Verification items for the finished model (mm, model axes). Face numbers are marked on the shaded views. A direction names the side the tool comes from. Give positions to 0.01 mm unless a question says otherwise; leave off trailing zeros. Order: outer loops, then holes, each group sorted by start corner. A loop starts at its lowest first (then second) coordinate and runs counter-clockwise, first axis right, second up.
from build123d import *

# Parameters (mm, degrees)
F1_DEPTH = 6.35


with BuildPart() as f1:
    # F0 (on Front) → F1 (new body)
    with BuildSketch(Plane.XZ):
        with BuildLine():
            ThreePointArc((11.4914766139, 0.1410518603), (11.4921258391, 0.0705272582), (11.4923422502, 0))
            ThreePointArc((11.4923422502, 0), (11.4921258391, -0.0705272582), (11.4914766139, -0.1410518603))
            Line((11.4914766139, -0.1410518603), (11.5924987112, 0))
            Line((11.5924987112, 0), (11.4914766139, 0.1410518603))
        make_face()
        with BuildLine():
            ThreePointArc((10.4146627839, 4.8588815063), (11.204205236, 2.5572867309), (11.4914766139, 0.1410518603))
            Line((11.4914766139, 0.1410518603), (11.5924987112, 0))
            Line((11.5924987112, 0), (13.8578264949, 3.1629584667))
            Line((13.8578264949, 3.1629584667), (10.44448044, 5.0297966865))
            Line((10.44448044, 5.0297966865), (10.4146627839, 4.8588815063))
        make_face()
        with BuildLine():
            Line((11.5924987112, 0), (11.4914766139, -0.1410518603))
            ThreePointArc((11.4914766139, -0.1410518603), (11.204205236, -2.5572867309), (10.4146627839, -4.8588815063))
            Line((10.4146627839, -4.8588815063), (10.44448044, -5.0297966865))
            Line((10.44448044, -5.0297966865), (13.8578264949, -3.1629584667))
            Line((13.8578264949, -3.1629584667), (11.5924987112, 0))
        make_face()
        with BuildLine():
            ThreePointArc((10.2922625668, 5.1130481761), (10.3542425867, 4.9863404267), (10.4146627839, 4.8588815063))
            Line((10.4146627839, 4.8588815063), (10.44448044, 5.0297966865))
            Line((10.44448044, 5.0297966865), (10.2922625668, 5.1130481761))
        make_face()
        with BuildLine():
            Line((10.44448044, -5.0297966865), (10.4146627839, -4.8588815063))
            ThreePointArc((10.4146627839, -4.8588815063), (10.3542425867, -4.9863404267), (10.2922625668, -5.1130481761))
            Line((10.2922625668, -5.1130481761), (10.44448044, -5.0297966865))
        make_face()
        with BuildLine():
            ThreePointArc((7.2750972621, 8.8964538004), (8.9850749785, 7.1653581925), (10.2922625668, 5.1130481761))
            Line((10.2922625668, 5.1130481761), (10.44448044, 5.0297966865))
            Line((10.44448044, 5.0297966865), (11.1131140025, 8.8624126846))
            Line((11.1131140025, 8.8624126846), (7.2278047245, 9.0633804529))
            Line((7.2278047245, 9.0633804529), (7.2750972621, 8.8964538004))
        make_face()
        with BuildLine():
            Line((10.44448044, -5.0297966865), (10.2922625668, -5.1130481761))
            ThreePointArc((10.2922625668, -5.1130481761), (8.9850749785, -7.1653581925), (7.2750972621, -8.8964538004))
            Line((7.2750972621, -8.8964538004), (7.2278047245, -9.0633804529))
            Line((7.2278047245, -9.0633804529), (11.1131140025, -8.8624126846))
            Line((11.1131140025, -8.8624126846), (10.44448044, -5.0297966865))
        make_face()
        with BuildLine():
            ThreePointArc((7.054539692, 9.0723425932), (7.1653581925, 8.9850749785), (7.2750972621, 8.8964538004))
            Line((7.2750972621, 8.8964538004), (7.2278047245, 9.0633804529))
            Line((7.2278047245, 9.0633804529), (7.054539692, 9.0723425932))
        make_face()
        with BuildLine():
            Line((7.2278047245, -9.0633804529), (7.2750972621, -8.8964538004))
            ThreePointArc((7.2750972621, -8.8964538004), (7.1653581925, -8.9850749785), (7.054539692, -9.0723425932))
            Line((7.054539692, -9.0723425932), (7.2278047245, -9.0633804529))
        make_face()
        with BuildLine():
            ThreePointArc((2.6946095043, 11.1719743114), (4.9863404267, 10.3542425867), (7.054539692, 9.0723425932))
            Line((7.054539692, 9.0723425932), (7.2278047245, 9.0633804529))
            Line((7.2278047245, 9.0633804529), (6.1673129885, 12.80655738))
            Line((6.1673129885, 12.80655738), (2.5795736401, 11.3018505655))
            Line((2.5795736401, 11.3018505655), (2.6946095043, 11.1719743114))
        make_face()
        with BuildLine():
            Line((7.2278047245, -9.0633804529), (7.054539692, -9.0723425932))
            ThreePointArc((7.054539692, -9.0723425932), (4.9863404267, -10.3542425867), (2.6946095043, -11.1719743114))
            Line((2.6946095043, -11.1719743114), (2.5795736401, -11.3018505655))
            Line((2.5795736401, -11.3018505655), (6.1673129885, -12.80655738))
            Line((6.1673129885, -12.80655738), (7.2278047245, -9.0633804529))
        make_face()
        with BuildLine():
            ThreePointArc((2.419578713, 11.2347482948), (2.5572867309, 11.204205236), (2.6946095043, 11.1719743114))
            Line((2.6946095043, 11.1719743114), (2.5795736401, 11.3018505655))
            Line((2.5795736401, 11.3018505655), (2.419578713, 11.2347482948))
        make_face()
        with BuildLine():
            Line((2.5795736401, -11.3018505655), (2.6946095043, -11.1719743114))
            ThreePointArc((2.6946095043, -11.1719743114), (2.5572867309, -11.204205236), (2.419578713, -11.2347482948))
            Line((2.419578713, -11.2347482948), (2.5795736401, -11.3018505655))
        make_face()
        with BuildLine():
            ThreePointArc((-2.419578713, 11.2347482948), (0, 11.4923422502), (2.419578713, 11.2347482948))
            Line((2.419578713, 11.2347482948), (2.5795736401, 11.3018505655))
            Line((2.5795736401, 11.3018505655), (0, 14.2142063241))
            Line((0, 14.2142063241), (-2.5795736401, 11.3018505655))
            Line((-2.5795736401, 11.3018505655), (-2.419578713, 11.2347482948))
        make_face()
        with BuildLine():
            Line((2.5795736401, -11.3018505655), (2.419578713, -11.2347482948))
            ThreePointArc((2.419578713, -11.2347482948), (0, -11.4923422502), (-2.419578713, -11.2347482948))
            Line((-2.419578713, -11.2347482948), (-2.5795736401, -11.3018505655))
            Line((-2.5795736401, -11.3018505655), (0, -14.2142063241))
            Line((0, -14.2142063241), (2.5795736401, -11.3018505655))
        make_face()
        with BuildLine():
            ThreePointArc((-2.6946095043, 11.1719743114), (-2.5572867309, 11.204205236), (-2.419578713, 11.2347482948))
            Line((-2.419578713, 11.2347482948), (-2.5795736401, 11.3018505655))
            Line((-2.5795736401, 11.3018505655), (-2.6946095043, 11.1719743114))
        make_face()
        with BuildLine():
            Line((-2.5795736401, -11.3018505655), (-2.419578713, -11.2347482948))
            ThreePointArc((-2.419578713, -11.2347482948), (-2.5572867309, -11.204205236), (-2.6946095043, -11.1719743114))
            Line((-2.6946095043, -11.1719743114), (-2.5795736401, -11.3018505655))
        make_face()
        with BuildLine():
            ThreePointArc((-7.054539692, 9.0723425932), (-4.9863404267, 10.3542425867), (-2.6946095043, 11.1719743114))
            Line((-2.6946095043, 11.1719743114), (-2.5795736401, 11.3018505655))
            Line((-2.5795736401, 11.3018505655), (-6.1673129885, 12.80655738))
            Line((-6.1673129885, 12.80655738), (-7.2278047245, 9.0633804529))
            Line((-7.2278047245, 9.0633804529), (-7.054539692, 9.0723425932))
        make_face()
        with BuildLine():
            Line((-2.5795736401, -11.3018505655), (-2.6946095043, -11.1719743114))
            ThreePointArc((-2.6946095043, -11.1719743114), (-4.9863404267, -10.3542425867), (-7.054539692, -9.0723425932))
            Line((-7.054539692, -9.0723425932), (-7.2278047245, -9.0633804529))
            Line((-7.2278047245, -9.0633804529), (-6.1673129885, -12.80655738))
            Line((-6.1673129885, -12.80655738), (-2.5795736401, -11.3018505655))
        make_face()
        with BuildLine():
            ThreePointArc((-7.2750972621, 8.8964538004), (-7.1653581925, 8.9850749785), (-7.054539692, 9.0723425932))
            Line((-7.054539692, 9.0723425932), (-7.2278047245, 9.0633804529))
            Line((-7.2278047245, 9.0633804529), (-7.2750972621, 8.8964538004))
        make_face()
        with BuildLine():
            Line((-7.2278047245, -9.0633804529), (-7.054539692, -9.0723425932))
            ThreePointArc((-7.054539692, -9.0723425932), (-7.1653581925, -8.9850749785), (-7.2750972621, -8.8964538004))
            Line((-7.2750972621, -8.8964538004), (-7.2278047245, -9.0633804529))
        make_face()
        with BuildLine():
            ThreePointArc((-10.2922625668, 5.1130481761), (-8.9850749785, 7.1653581925), (-7.2750972621, 8.8964538004))
            Line((-7.2750972621, 8.8964538004), (-7.2278047245, 9.0633804529))
            Line((-7.2278047245, 9.0633804529), (-11.1131140025, 8.8624126846))
            Line((-11.1131140025, 8.8624126846), (-10.44448044, 5.0297966865))
            Line((-10.44448044, 5.0297966865), (-10.2922625668, 5.1130481761))
        make_face()
        with BuildLine():
            Line((-7.2278047245, -9.0633804529), (-7.2750972621, -8.8964538004))
            ThreePointArc((-7.2750972621, -8.8964538004), (-8.9850749785, -7.1653581925), (-10.2922625668, -5.1130481761))
            Line((-10.2922625668, -5.1130481761), (-10.44448044, -5.0297966865))
            Line((-10.44448044, -5.0297966865), (-11.1131140025, -8.8624126846))
            Line((-11.1131140025, -8.8624126846), (-7.2278047245, -9.0633804529))
        make_face()
        with BuildLine():
            ThreePointArc((-10.4146627839, 4.8588815063), (-10.3542425867, 4.9863404267), (-10.2922625668, 5.1130481761))
            Line((-10.2922625668, 5.1130481761), (-10.44448044, 5.0297966865))
            Line((-10.44448044, 5.0297966865), (-10.4146627839, 4.8588815063))
        make_face()
        with BuildLine():
            Line((-10.44448044, -5.0297966865), (-10.2922625668, -5.1130481761))
            ThreePointArc((-10.2922625668, -5.1130481761), (-10.3542425867, -4.9863404267), (-10.4146627839, -4.8588815063))
            Line((-10.4146627839, -4.8588815063), (-10.44448044, -5.0297966865))
        make_face()
        with BuildLine():
            ThreePointArc((-11.4914766139, 0.1410518603), (-11.204205236, 2.5572867309), (-10.4146627839, 4.8588815063))
            Line((-10.4146627839, 4.8588815063), (-10.44448044, 5.0297966865))
            Line((-10.44448044, 5.0297966865), (-13.8578264949, 3.1629584667))
            Line((-13.8578264949, 3.1629584667), (-11.5924987112, 0))
            Line((-11.5924987112, 0), (-11.4914766139, 0.1410518603))
        make_face()
        with BuildLine():
            Line((-10.44448044, -5.0297966865), (-10.4146627839, -4.8588815063))
            ThreePointArc((-10.4146627839, -4.8588815063), (-11.204205236, -2.5572867309), (-11.4914766139, -0.1410518603))
            Line((-11.4914766139, -0.1410518603), (-11.5924987112, 0))
            Line((-11.5924987112, 0), (-13.8578264949, -3.1629584667))
            Line((-13.8578264949, -3.1629584667), (-10.44448044, -5.0297966865))
        make_face()
        with BuildLine():
            ThreePointArc((-11.4914766139, -0.1410518603), (-11.4923422502, 0), (-11.4914766139, 0.1410518603))
            Line((-11.4914766139, 0.1410518603), (-11.5924987112, 0))
            Line((-11.5924987112, 0), (-11.4914766139, -0.1410518603))
        make_face()
    extrude(amount=F1_DEPTH)


solid = f1.part
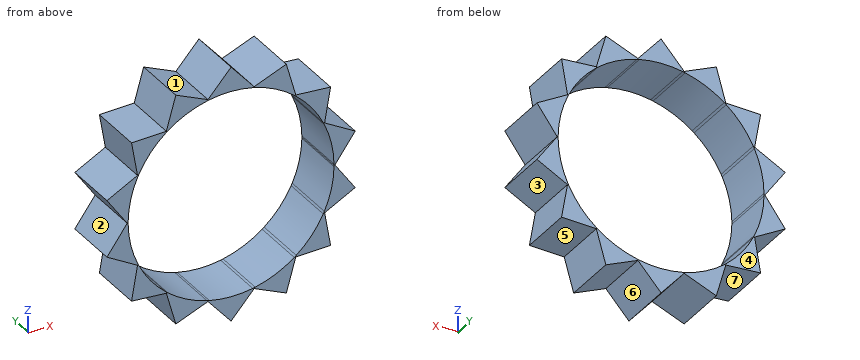
(1) Section check A-A, the plane x = -0.5. Enter the section's corners in (y, z), then the cut area to 3 significant figures.
Solved:
outline: (-6.35, -13.65) - (0, -13.65) - (0, -11.48) - (-6.35, -11.48) - close; (-6.35, 11.48) - (0, 11.48) - (0, 13.65) - (-6.35, 13.65) - close
area: 27.5 mm2
(2) Release check for a two-part mould opening along X. For the marked faces 4, 5, 6 and 7 record: pulls with the +X half, pulls with the -X half, needs draft (parallel to the pull), parting line crosses it, or undercut.
Solved:
face 4: needs draft
face 5: pulls with the +X half
face 6: undercut
face 7: pulls with the -X half
(3) Scan lines: line 1 (X direction, y = -3.25, z = 12.25) (3 decimals); line 2 (Z direction, x = -4, y = -3); line 3 (X direction, y = -2.25, z = -10.5). Record each from-to range of solid material in increasing order.
Solved:
line 1: x = -6.325 to -4.84, -1.74 to 1.74, 4.84 to 6.325
line 2: z = -11.9 to -10.77, 10.77 to 11.9
line 3: x = -6.82 to -4.67, 4.67 to 6.82
(4) Set-up check for the marked faces 1, 2 and 3: record each of +Z, -Z, +X, -X, +Y, -Y from which the full face is reachable in a straight line by a thin tool's end or side.
Solved:
face 1: +Z, +Y, -Y
face 2: -X, +Y, -Y
face 3: +X, +Y, -Y
(5) Section check B-B, the plane z = -7.75. Enter the section's corners in (x, y).
Solved:
outline: (-10.92, -6.35) - (-8.49, -6.35) - (-8.49, 0) - (-10.92, 0) - close; (8.49, -6.35) - (10.92, -6.35) - (10.92, 0) - (8.49, 0) - close
(6) Section check C-C, the plane z = 12.25. Enter the section's corners in (x, y) (3 decimals), then the cut area to 3 significant figures.
Solved:
outline: (-6.325, -6.35) - (-4.84, -6.35) - (-4.84, 0) - (-6.325, 0) - close; (-1.74, -6.35) - (1.74, -6.35) - (1.74, 0) - (-1.74, 0) - close; (4.84, -6.35) - (6.325, -6.35) - (6.325, 0) - (4.84, 0) - close
area: 41.0 mm2
(7) Go/stop test with flat-tipped pins: pin 1 (3 mm diameter, centred on y = -5, z = 1.5, fed in from +X); pin 2 (1 mm diameter, centred on x = 8, y = -1.5, fed in from -Z). Record where each tip stops, or that it passes through.
Solved:
pin 1: stops at x = 13.74
pin 2: stops at z = -9.05
